from build123d import *

# Parameters (mm, degrees)
ESBO_O1_R                = 2
ESBO_O1_W                = 6
ESBO_O1_H                = 1.5
RESSALTO_EXTRUS_O1_DEPTH = 10
RESSALTO_EXTRUS_O4_START = -4
RESSALTO_EXTRUS_O4_DEPTH = 8
CORTE_EXTRUS_O1_START    = -5.890675
ESBO_O3_W                = 6
ESBO_O3_H                = 3
CORTE_EXTRUS_O1_DEPTH    = 9.890675


with BuildPart() as part:
    # Esboço1 → Ressalto-extrusão1 (new body)
    with BuildSketch(Plane.XY):
        with BuildLine():
            Line((-28, -7), (-22, -7))
            Line((-22, -7), (-22, -13.2))
            Line((-22, -13.2), (-28, -13.2))
            Line((-28, -13.2), (-28, -15.2))
            Line((-28, -15.2), (-20, -15.2))
            Line((-20, -15.2), (-20, -14.1))
            Line((-20, -14.1), (1.739413567, -3.602005059))
            ThreePointArc((1.739413567, -3.602005059), (3.388041784, -2.12630498), (4, 0))
            Line((4, 0), (4, 8))
            Line((4, 8), (-4, 8))
            Line((-4, 8), (-4, 2.403900213))
            Line((-4, 2.403900213), (-20, -6.1))
            Line((-20, -6.1), (-20, -5))
            Line((-20, -5), (-28, -5))
            Line((-28, -5), (-28, -7))
        make_face()
        Circle(ESBO_O1_R, mode=Mode.SUBTRACT)
        with Locations((0, 6.55)):
            Rectangle(ESBO_O1_W, ESBO_O1_H, mode=Mode.SUBTRACT)
    extrude(amount=RESSALTO_EXTRUS_O1_DEPTH)

    # Esboço2 → Ressalto-extrusão4 (add)
    with BuildSketch(Plane(origin=(0, 0, 0), x_dir=(0, 0, -1), z_dir=(1, 0, 0)).offset(RESSALTO_EXTRUS_O4_START)):
        with BuildLine():
            ThreePointArc((-10, 9.543560763), (-5, 8.5), (0, 9.543560763))
            Line((0, 9.543560763), (0, 8))
            Line((0, 8), (-10, 8))
            Line((-10, 8), (-10, 9.543560763))
        make_face()
    extrude(amount=RESSALTO_EXTRUS_O4_DEPTH)

    # Esboço3 → Corte-extrusão1 (cut)
    with BuildSketch(Plane(origin=(0, 0, 0), x_dir=(1, 0, 0), z_dir=(0, 1, 0)).offset(CORTE_EXTRUS_O1_START)):
        with Locations((0, -5)):
            Rectangle(ESBO_O3_W, ESBO_O3_H)
    extrude(amount=CORTE_EXTRUS_O1_DEPTH, mode=Mode.SUBTRACT)


solid = part.part
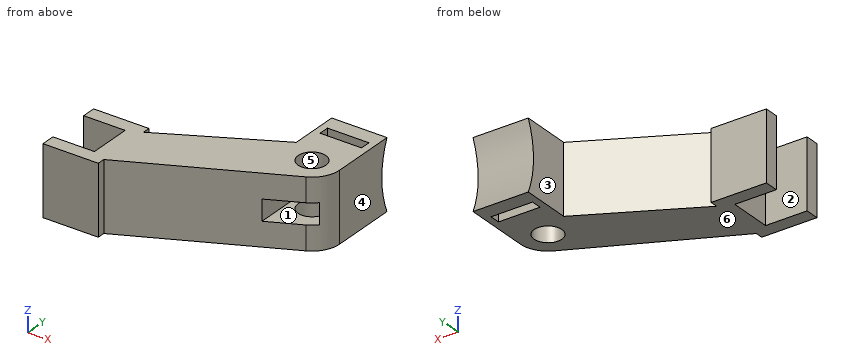
Work out the finished part from the listing and answer in its coordinate system (mm). Face numbers are marked on the shaded views. A direction names the side the tool comes from. Coordinates: 2 decimals unless noted, no trailing zeros. Write each loop counter-clockwise with the first axis right and the second up, starting at its lowest first coordinate (ties: lowest second). Pieces come first, ordered by that corner, then holes. Notation, with made-up numbers: M -6.75,-19 L 1.25,-19 A22 cw 1.25,1 Z; hole C -15,15 d9. An arc over 180 degrees is marked long. Answer as CSV lines item,"result". Start each with the question number.
Item 1: Consider L1, parallel to Y at x = 0, z = 9.2; L2, parallel to Y at x = -24, z = 4.75; L3, parallel to Y at x = 0, z = 2.25. Determine where each line is inside the solid, lowest interval first.
Item 2: Determine the mould class of the marked faces 4, 5 and 6 for opening direction X: released by +X, released by -X, zero draft, split by the parting line, or undercut.
Item 3: A tool of negligible diameter and unlimited length cuts with its end or side. For the marked faces 1, 2 and 3, from which of +Z, -Z, +X, -X, +Y, -Y can it reach the whole face along a straight path? Write none if from no direction.
Item 4: Section B-B on y = -5.5 is taken. Write down the section's boundary in (x, z).
Item 5: Section D-D on z = 9.5 is taken. Write down the section's boundary in (x, y).
Item 6: Section A-A on z = 5 is taken. Write down the section's boundary in (x, y).
Item 7: Flat-ended cylindrical pins translate along their axes: P1, Ø4, axis at x = -24, z = 4, coming from the +Y side; P2, Ø1, axis at y = -9, z = 8, coming from the -X side; P3, Ø5, axis at x = 1, z = 3.5, coming from the -Y side. Find the tip coordinate at first contact, or state that the pin passes through.
Item 8: Section C-C on x = 0 is taken. Write down the section's boundary in (y, z), and give its area (3 significant figures).
Checks:
1,L1,"y = -4.44 to -2, 2 to 5.8, 7.3 to 9.23"
1,L2,"y = -15.2 to -13.2, -7 to -5"
1,L3,"y = -4.44 to -2, 2 to 5.8, 7.3 to 8.81"
2,face 4,"released by +X"
2,face 5,"undercut"
2,face 6,"zero draft"
3,face 1,"-Y"
3,face 2,"+Z, -Z, -X"
3,face 3,"+Z, -Z, -X, +Y"
4,outline,"M -28,0 L -20,0 L -20,10 L -28,10 Z; M -18.87,0 L -2.19,0 L -2.19,3.5 L -3,3.5 L -3,6.5 L -2.19,6.5 L -2.19,10 L -18.87,10 Z"
5,outline,"M -28,-15.2 L -20,-15.2 L -20,-14.1 L 1.74,-3.6 A4 ccw 4,0 L 4,9.34 L -4,9.34 L -4,2.4 L -20,-6.1 L -20,-5 L -28,-5 L -28,-7 L -22,-7 L -22,-13.2 L -28,-13.2 Z; hole M -3,5.8 L 3,5.8 L 3,7.3 L -3,7.3 Z; hole C 0,0 d4"
6,outline,"M -28,-15.2 L -20,-15.2 L -20,-14.1 L -3,-5.89 L -3,4 L 3,4 L 3,-2.65 A4 ccw 4,0 L 4,8.5 L -4,8.5 L -4,2.4 L -20,-6.1 L -20,-5 L -28,-5 L -28,-7 L -22,-7 L -22,-13.2 L -28,-13.2 Z; hole M -3,5.8 L 3,5.8 L 3,7.3 L -3,7.3 Z"
7,P1,"stops at y = -5"
7,P2,"stops at x = -22"
7,P3,"stops at y = -5.17"
8,outline,"M -4.44,0 L -2,0 L -2,3.5 L -4.44,3.5 Z; M -4.44,6.5 L -2,6.5 L -2,10 L -4.44,10 Z; M 2,0 L 5.8,0 L 5.8,10 L 2,10 L 2,6.5 L 4,6.5 L 4,3.5 L 2,3.5 Z; M 7.3,0 L 9.54,0 A12.5 cw 9.54,10 L 7.3,10 Z"
8,area,"64.5 mm²"
